Input: dimensioned drawing with shaded views. Units: mm. Origin: part minimum x, y, z. Coordinates: 2 decimals unless noted, no trailing zeros. Order: outer loops, then holes, each group sorted by start corner. A loop starts at its lowest first (then second) coordinate and runs counter-clockwise, first axis right, second up. Notation, with made-up numbers: M 53.25,-4.75 L 77.25,-4.75 A20 ccw 77.25,8.25 Z; hole C -7,-5.75 d5. An arc over 180 degrees is marked long. Use CSV: the item, a comma, the result in double quotes. Start each with the question number.
1. Section query C-C on y = 3.25. Return the cut outline in (x, z).
2. Section query B-B on z = 16. Return the cut outline in (x, y).
3. Section query A-A on x = 0.45. Return the cut outline in (y, z).
4. First-contact query: P1, Ø0.5, axis at x = 1, y = 0.5, coming from the -Z side; P2, Ø0.8, axis at x = 0.5, z = 32.5, coming from the +Y side; P3, Ø0.8, axis at x = 0.5, y = 0.5, coming from the +Z side. Flat tips, straight axial feed; report the tip coordinate or a pass-through.
5. Section query D-D on z = 4. Return the cut outline in (x, y).
6. Material intervals for line 1 (Z direction, x = 0.15, y = 6.5); line 2 (Z direction, x = 0.8, y = 9); line 3 (Y direction, x = 1.25, z = 15.5) (1 decimal), sorted ascending.
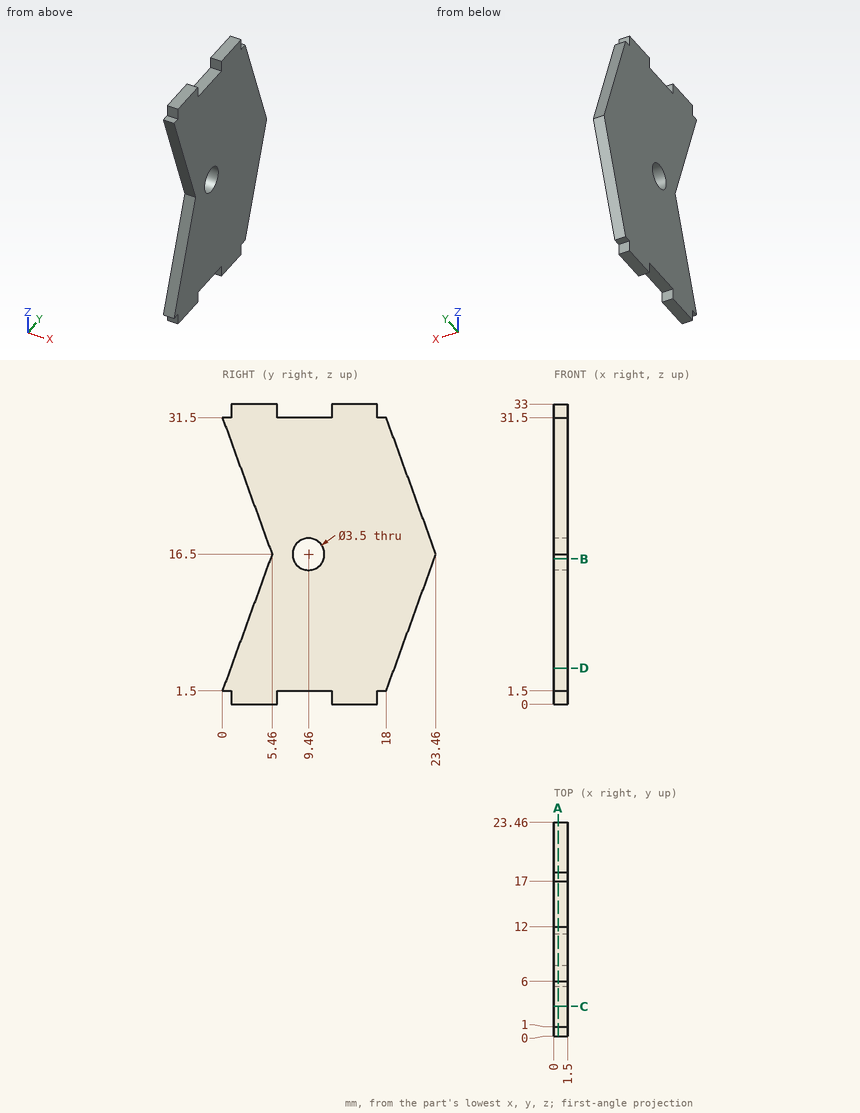
Results list:
1,outline,"M 0,0 L 1.5,0 L 1.5,10.43 L 0,10.43 Z; M 0,22.57 L 1.5,22.57 L 1.5,33 L 0,33 Z"
2,outline,"M 0,5.28 L 1.5,5.28 L 1.5,7.78 L 0,7.78 Z; M 0,11.14 L 1.5,11.14 L 1.5,23.28 L 0,23.28 Z"
3,outline,"M 0,1.5 L 1,1.5 L 1,0 L 6,0 L 6,1.5 L 12,1.5 L 12,0 L 17,0 L 17,1.5 L 18,1.5 L 23.46,16.5 L 18,31.5 L 17,31.5 L 17,33 L 12,33 L 12,31.5 L 6,31.5 L 6,33 L 1,33 L 1,31.5 L 0,31.5 L 5.46,16.5 Z; hole C 9.46,16.5 d3.5"
4,P1,"stops at z = 1.5"
4,P2,"stops at y = 17"
4,P3,"stops at z = 31.5"
5,outline,"M 0,0.91 L 1.5,0.91 L 1.5,18.91 L 0,18.91 Z"
6,line 1,"z = 1.5 to 31.5"
6,line 2,"z = 1.5 to 14.81, 18.19 to 31.5"
6,line 3,"y = 5.1 to 8, 10.9 to 23.1"
